from build123d import *

# Parameters (mm, degrees)
SKETCH1_W           = 100
SKETCH1_H           = 90
BOSS_EXTRUDE1_DEPTH = 6
SKETCH2_R           = 2.75
SKETCH2_R_2         = 3.25
CUT_EXTRUDE1_DEPTH  = 68.53517602
SKETCH3_W           = 42
SKETCH3_H           = 42
CUT_EXTRUDE2_DEPTH  = 10


with BuildPart() as part:
    # Sketch1 → Boss-Extrude1 (new body)
    with BuildSketch(Plane.XY):
        Rectangle(SKETCH1_W, SKETCH1_H)
    extrude(amount=BOSS_EXTRUDE1_DEPTH)

    # Sketch2 → Cut-Extrude1 (cut, through all)
    with BuildSketch(Plane.XY.offset(6)):
        with Locations((-25, 0)):
            Circle(SKETCH2_R)
        with Locations((-42, 30)):
            Circle(SKETCH2_R_2)
        with Locations(Location((-42, -30, 0), (0, 0, 180))):
            Circle(SKETCH2_R_2)
        with Locations((42, -30)):
            Circle(SKETCH2_R_2)
        with Locations(Location((25, 0, 0), (0, 0, 180))):
            Circle(SKETCH2_R)
        with Locations(Location((42, 30, 0), (0, 0, 180))):
            Circle(SKETCH2_R_2)
    extrude(amount=-CUT_EXTRUDE1_DEPTH, mode=Mode.SUBTRACT)

    # Sketch3 → Cut-Extrude2 (cut)
    with BuildSketch(Plane.XY.offset(6)):
        Rectangle(SKETCH3_W, SKETCH3_H)
    extrude(amount=-CUT_EXTRUDE2_DEPTH, mode=Mode.SUBTRACT)


solid = part.part
Here's how the part is built. I have some questions about the finished solid (model axes, mm). A direction names the side the tool comes from. Coordinates: 2 decimals unless noted, no trailing zeros. Loops run counter-clockwise (first coordinate to the right, second up) from the corner with the lowest first, then second, coordinate; pieces in that order, holes last.
1. Imagine slicing it at B-B, the plane z = 3.2. Please give me the cut outline in (x, y).
2. For faces 5 (the flat face through (0, -21, 3)), 6 (the flat face through (-50, -1, 3)), which set-ups out of +Z, -Z, +X, -X, +Y, -Y let a thin tool reach every point of the face, with its end or its side?
3. Imagine slicing it at D-D, the plane x = 25. Please give me the cut outline in (y, z), and give its area (3 significant figures).
4. For P1, Ø4, axis at x = -42, y = -30, coming from the -Z side; P2, Ø5, axis at x = 22.5, y = 4, coming from the -Z side, each with a flat end and sliding along its axis, tell me the tip position at first contact or that it passes through.
5. Imagine slicing it at A-A, the plane y = -30. Please give me the cut outline in (x, z).
6. I need wall thicknesses on L1, parallel to Y at x = 42, z = 1.2; L2, parallel to Y at x = 13, z = 1.4; L3, parallel to Y at x = 25, z = 4.15. Which ranges of each line are inside material? Lowest first, please.
7. Imagine slicing it at C-C, the plane x = -42. Please give me the cut outline in (y, z).
8. If we mould it in two halves opening along Y, with no side actions, what happens to faces 1 (the cylindrical face through (45.002, -31.245, 3.042)), 2 (the flat face through (22, 1, 0)), 3 (the flat face through (-1, -45, 3)), 4 (the flat face through (0, 21, 3))? For each: pulls with the +Y half, pulls with the -Y half, needs draft (parallel to the pull), parting line crosses it, or undercut.
Taken from the geometry:
1. outline: (-50, -45) - (50, -45) - (50, 45) - (-50, 45) - close; hole circle Ø6.5 at (-42, -30); hole circle Ø6.5 at (-42, 30); hole circle Ø5.5 at (-25, 0); hole (-21, -21) - (21, -21) - (21, 21) - (-21, 21) - close; hole circle Ø5.5 at (25, 0); hole circle Ø6.5 at (42, -30); hole circle Ø6.5 at (42, 30)
2. face 5: +Z, -Z
2. face 6: +Z, -Z, -X, +Y, -Y
3. outline: (-45, 0) - (-2.75, 0) - (-2.75, 6) - (-45, 6) - close; (2.75, 0) - (45, 0) - (45, 6) - (2.75, 6) - close
3. area: 507 mm2
4. P1: passes through
4. P2: stops at z = 0
5. outline: (-50, 0) - (-45.25, 0) - (-45.25, 6) - (-50, 6) - close; (-38.75, 0) - (38.75, 0) - (38.75, 6) - (-38.75, 6) - close; (45.25, 0) - (50, 0) - (50, 6) - (45.25, 6) - close
6. L1: y = -45 to -33.25, -26.75 to 26.75, 33.25 to 45
6. L2: y = -45 to -21, 21 to 45
6. L3: y = -45 to -2.75, 2.75 to 45
7. outline: (-45, 0) - (-33.25, 0) - (-33.25, 6) - (-45, 6) - close; (-26.75, 0) - (26.75, 0) - (26.75, 6) - (-26.75, 6) - close; (33.25, 0) - (45, 0) - (45, 6) - (33.25, 6) - close
8. face 1: undercut
8. face 2: needs draft
8. face 3: pulls with the -Y half
8. face 4: undercut
